Autodesk Inventor part; units mm, degrees
ref_plane "YZ Plane" through (0, 0, 0) normal (1, 0, 0) x (0, 1, 0)
ref_plane "XZ Plane" through (0, 0, 0) normal (0, 1, 0) x (-1, 0, 0)
ref_plane "XY Plane" through (0, 0, 0) normal (0, 0, 1) x (1, 0, 0)
sketch "スケッチ1" plane through (0, 0, 0) normal (0, 0, 1) x (1, 0, 0)
  circle A0 centre (0, 0) radius 18
  dimension "d0" = 36
extrude "押し出し1" add sketch "スケッチ1" along normal blind 4.25
sketch "スケッチ2" plane through (0, 0, 4.25) normal (0, 0, 1) x (1, 0, 0)
  circle A0 centre (0, 0) radius 6
  point P0 (0, 6)
  point P1 (-6, 0)
  point P2 (0, -6)
  point P3 (6, 0)
  dimension "d3" = 12
  dimension "d6" = 360
hole "穴1" at (0, 6, 4.25) at (-6, 0, 4.25) at (0, -6, 4.25) at (6, 0, 4.25) direction (0, 0, -1) diameter 3.2 end through all
sketch "スケッチ3" plane through (0, 0, 0) normal (0, 0, -1) x (-1, 0, 0)
  circle A0 centre (0, 0) radius 8.5
  point P0 (-6.0104, 6.0104)
  point P1 (-6.0104, -6.0104)
  point P2 (6.0104, -6.0104)
  point P3 (6.0104, 6.0104)
  dimension "d15" = 17
  dimension "d18" = 360
hole "穴2" at (6.0104, 6.0104, 0) at (6.0104, -6.0104, 0) at (-6.0104, -6.0104, 0) at (-6.0104, 6.0104, 0) direction (0, 0, 1) diameter 3.2 end through all counterbore diameter 6.5 counterbore depth 10
sketch "スケッチ4" plane through (0, 0, 0) normal (0, 0, -1) x (-1, 0, 0)
  circle A0 centre (0, 0) radius 3.25
  dimension "d27" = 6.5
extrude "押し出し2" cut sketch "スケッチ4" against normal blind 8
sketch "スケッチ5" plane through (0, 0, 4.25) normal (0, 0, 1) x (1, 0, 0)
  circle A0 centre (0, 0) radius 15
  point P0 (0, -15)
  point P1 (10.6066, -10.6066)
  point P2 (15, 0)
  point P3 (10.6066, 10.6066)
  point P4 (0, 15)
  point P5 (-10.6066, 10.6066)
  point P6 (-15, 0)
  point P7 (-10.6066, -10.6066)
  dimension "d31" = 30
  dimension "d34" = 360
hole "穴3" at (0, -15, 4.25) at (10.6066, -10.6066, 4.25) at (15, 0, 4.25) at (10.6066, 10.6066, 4.25) at (0, 15, 4.25) at (-10.6066, 10.6066, 4.25) at (-15, 0, 4.25) at (-10.6066, -10.6066, 4.25) direction (0, 0, -1) diameter 3.2 end through all
sketch "スケッチ6" plane through (0, 0, 4.25) normal (0, 0, -1) x (-1, 0, 0)
  circle A0 centre (0, 0) radius 12
  dimension "d43" = 24
extrude "押し出し3" cut sketch "スケッチ6" along normal blind 1
properties part number "s_base6"
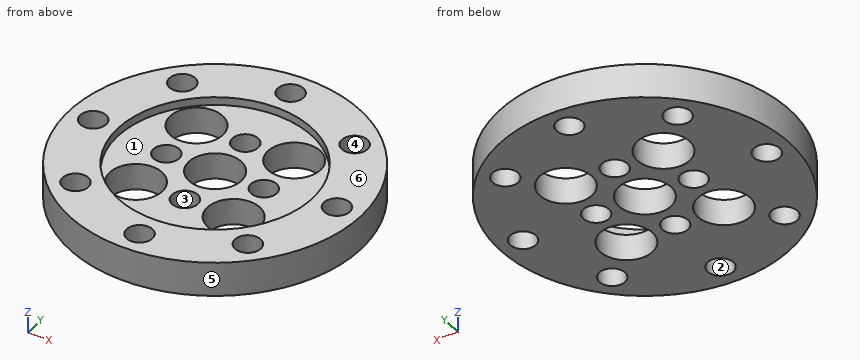
Source: CAD feature listing. Evaluate the final solid. Frame: model axes, mm. Face numbers are marked on the shaded views. A direction names the side the tool comes from. Round coordinates to 2 decimals unless told otherwise and drop trailing zeros. Loops run counter-clockwise (first coordinate to the right, second up) from the corner with the lowest first, then second, coordinate; pieces in that order, holes last. Notation, with made-up numbers: M 9,81 L 53,81 A20 cw 53,92 Z; hole C 5.5,-2.75 d5. An arc over 180 degrees is marked long. Return JSON: item names as keys, results as strings. Group by question number.
1. Section query B-B on x = -15. Output: boundary loops of the cut face in (y, z).
2. Pin query (flat end, axial travel): pin 1 (6 mm diameter, centred on x = -6.01, y = -6.01, fed in from -Z). Return the tip coordinate at first contact, or that it passes through.
3. Material intervals for line 1 along Y through (x, z) = (0, 1.65); line 2 along X through (y, z) = (-9.5, 3.2); line 3 along X through (y, z) = (5, 1.95), sorted ascending. Write a range as from..to.
4. Section query A-A on y = 0. Output: boundary loops of the cut face in (x, z), and give its area (3 significant figures).
5. Mould query, pull axis Y, two halves, no side actions, for the marked faces 3, 4, 5 and 6. Classes: released by +Y, released by -Y, zero draft, split by the parting line, or undercut.
6. Section query D-D on y = 10. Output: boundary loops of the cut face in (x, z).
7. Reachability of the marked faces 1 and 2 from +Z, -Z, +X, -X, +Y, -Y: full face, straight path, thin tool, end or side. Return the list, or none.
8. Section query C-C on y = 14. Output: boundary loops of the cut face in (x, z).
Checks:
{
 "1": {"outline": "M -9.95,0 L -1.6,0 L -1.6,4.25 L -9.95,4.25 Z; M 1.6,0 L 9.95,0 L 9.95,4.25 L 1.6,4.25 Z"},
 "2": {"pin 1": "passes through"},
 "3": {"line 1": "y = -18..-16.6, -13.4..-7.6, -4.4..-3.25, 3.25..4.4, 7.6..13.4, 16.6..18", "line 2": "x = -15.29..-11.76, -9.45..9.45, 11.76..15.29", "line 3": "x = -17.29..-9.1, -2.92..-1.25, 1.25..2.92, 9.1..17.29"},
 "4": {"outline": "M -18,0 L -16.6,0 L -16.6,4.25 L -18,4.25 Z; M -13.4,0 L -7.6,0 L -7.6,3.25 L -12,3.25 L -12,4.25 L -13.4,4.25 Z; M -4.4,0 L -3.25,0 L -3.25,3.25 L -4.4,3.25 Z; M 3.25,0 L 4.4,0 L 4.4,3.25 L 3.25,3.25 Z; M 7.6,0 L 13.4,0 L 13.4,4.25 L 12,4.25 L 12,3.25 L 7.6,3.25 Z; M 16.6,0 L 18,0 L 18,4.25 L 16.6,4.25 Z", "area": "59.9 mm²"},
 "5": {"face 3": "undercut", "face 4": "undercut", "face 5": "split by the parting line", "face 6": "zero draft"},
 "6": {"outline": "M -14.97,0 L -12.09,0 L -12.09,4.25 L -14.97,4.25 Z; M -9.13,0 L 9.13,0 L 9.13,4.25 L 6.63,4.25 L 6.63,3.25 L -6.63,3.25 L -6.63,4.25 L -9.13,4.25 Z; M 12.09,0 L 14.97,0 L 14.97,4.25 L 12.09,4.25 Z"},
 "7": {"face 1": "+Z", "face 2": "+Z, -Z"},
 "8": {"outline": "M -11.31,0 L -1.25,0 L -1.25,4.25 L -11.31,4.25 Z; M 1.25,0 L 11.31,0 L 11.31,4.25 L 1.25,4.25 Z"}
}
